The model under review builds one solid part; all positions refer to its coordinate system, in mm. Face numbers are marked on the shaded views. A direction names the side the tool comes from. Give positions to 0.01 mm unless a question says otherwise; leave off trailing zeros. Order: outer loops, then holes, each group sorted by start corner. A loop starts at its lowest first (then second) coordinate and runs counter-clockwise, first axis right, second up.
```python
from build123d import *

# Parameters (mm, degrees)
SKETCH_1_W          = 40
SKETCH_1_H          = 22
SKETCH_1_R          = 4.5
EXTRUDE_1_DEPTH     = 6
CUT_EXTRUDE_2_DEPTH = 4
SKETCH_4_R          = 4.5
CUT_EXTRUDE_3_DEPTH = 7
EXTRUDE_2_DEPTH     = 40
SKETCH_6_W          = 23
SKETCH_6_H          = 13
CUT_EXTRUDE_4_DEPTH = 40
SKETCH_7_R          = 1
CUT_EXTRUDE_5_DEPTH = 40


with BuildPart() as part:
    # 草图1 → 凸台-拉伸1 (new body)
    with BuildSketch(Plane.XY):
        Rectangle(SKETCH_1_W, SKETCH_1_H)
        with BuildLine():
            add(Edge.make_bspline(
                [(3.991210712, -4.387982431), (18, -3.591602336), (18, 0), (18, 3.591602336), (3.991210712, 4.387982431)],
                knots=[4.935981285, 4.935981285, 4.935981285, 6.283185307, 6.283185307, 7.630389329, 7.630389329, 7.630389329], degree=2, weights=[1, 0.781579788, 1, 0.781579788, 1]))
            add(Edge.make_bspline(
                [(3.991210712, 4.387982431), (0, 20.567539049), (-3.991210712, 4.387982431)],
                knots=[5.192517184, 5.192517184, 5.192517184, 7.373853431, 7.373853431, 7.373853431], degree=2, weights=[1, 0.461892887, 1]))
            add(Edge.make_bspline(
                [(-3.991210712, 4.387982431), (-18, 3.591602336), (-18, 0), (-18, -3.591602336), (-3.991210712, -4.387982431)],
                knots=[1.794388632, 1.794388632, 1.794388632, 3.141592654, 3.141592654, 4.488796676, 4.488796676, 4.488796676], degree=2, weights=[1, 0.781579788, 1, 0.781579788, 1]))
            add(Edge.make_bspline(
                [(-3.991210712, -4.387982431), (0, -20.567539049), (3.991210712, -4.387982431)],
                knots=[2.05092453, 2.05092453, 2.05092453, 4.232260777, 4.232260777, 4.232260777], degree=2, weights=[1, 0.461892887, 1]))
        make_face(mode=Mode.SUBTRACT)
        with BuildLine():
            add(Edge.make_bspline(
                [(-3.991210712, -4.387982431), (0, -20.567539049), (3.991210712, -4.387982431)],
                knots=[2.05092453, 2.05092453, 2.05092453, 4.232260777, 4.232260777, 4.232260777], degree=2, weights=[1, 0.461892887, 1]))
            add(Edge.make_bspline(
                [(3.991210712, -4.387982431), (18, -3.591602336), (18, 0), (18, 3.591602336), (3.991210712, 4.387982431)],
                knots=[4.935981285, 4.935981285, 4.935981285, 6.283185307, 6.283185307, 7.630389329, 7.630389329, 7.630389329], degree=2, weights=[1, 0.781579788, 1, 0.781579788, 1]))
            add(Edge.make_bspline(
                [(3.991210712, 4.387982431), (0, 20.567539049), (-3.991210712, 4.387982431)],
                knots=[5.192517184, 5.192517184, 5.192517184, 7.373853431, 7.373853431, 7.373853431], degree=2, weights=[1, 0.461892887, 1]))
            add(Edge.make_bspline(
                [(-3.991210712, 4.387982431), (-18, 3.591602336), (-18, 0), (-18, -3.591602336), (-3.991210712, -4.387982431)],
                knots=[1.794388632, 1.794388632, 1.794388632, 3.141592654, 3.141592654, 4.488796676, 4.488796676, 4.488796676], degree=2, weights=[1, 0.781579788, 1, 0.781579788, 1]))
        make_face()
        Circle(SKETCH_1_R, mode=Mode.SUBTRACT)
        Circle(SKETCH_1_R)
    extrude(amount=EXTRUDE_1_DEPTH)

    # 草图3 → 切除-拉伸2 (cut)
    with BuildSketch(Plane.XY.offset(6)):
        with BuildLine():
            add(Edge.make_bspline(
                [(3.991210712, -4.387982431), (18, -3.591602336), (18, 0), (18, 3.591602336), (3.991210712, 4.387982431)],
                knots=[4.935981285, 4.935981285, 4.935981285, 6.283185307, 6.283185307, 7.630389329, 7.630389329, 7.630389329], degree=2, weights=[1, 0.781579788, 1, 0.781579788, 1]))
            add(Edge.make_bspline(
                [(3.991210712, 4.387982431), (0, 20.567539049), (-3.991210712, 4.387982431)],
                knots=[5.192517184, 5.192517184, 5.192517184, 7.373853431, 7.373853431, 7.373853431], degree=2, weights=[1, 0.461892887, 1]))
            add(Edge.make_bspline(
                [(-3.991210712, 4.387982431), (-18, 3.591602336), (-18, 0), (-18, -3.591602336), (-3.991210712, -4.387982431)],
                knots=[1.794388632, 1.794388632, 1.794388632, 3.141592654, 3.141592654, 4.488796676, 4.488796676, 4.488796676], degree=2, weights=[1, 0.781579788, 1, 0.781579788, 1]))
            add(Edge.make_bspline(
                [(-3.991210712, -4.387982431), (0, -20.567539049), (3.991210712, -4.387982431)],
                knots=[2.05092453, 2.05092453, 2.05092453, 4.232260777, 4.232260777, 4.232260777], degree=2, weights=[1, 0.461892887, 1]))
        make_face()
    extrude(amount=-CUT_EXTRUDE_2_DEPTH, mode=Mode.SUBTRACT)

    # 草图4 → 切除-拉伸3 (cut, through all)
    with BuildSketch(Plane.XY.offset(6)):
        Circle(SKETCH_4_R)
    extrude(amount=-CUT_EXTRUDE_3_DEPTH, mode=Mode.SUBTRACT)

    # 草图5 → 凸台-拉伸2 (add)
    with BuildSketch(Plane.XY.offset(6)):
        Polygon((20, -11), (-20, -11), (-20, -9.5), (-20, 9.5), (-20, 11), (20, 11), (20, 9.5), (-18, 9.5), (-18, -9.5), (20, -9.5), align=None)
    extrude(amount=EXTRUDE_2_DEPTH)

    # 草图6 → 切除-拉伸4 (cut)
    with BuildSketch(Plane.ZY.offset(20)):
        with Locations((23, 0)):
            Rectangle(SKETCH_6_W, SKETCH_6_H)
    extrude(amount=-CUT_EXTRUDE_4_DEPTH, mode=Mode.SUBTRACT)

    # 草图7 → 切除-拉伸5 (cut)
    with BuildSketch(Plane.ZY.offset(20)):
        with Locations((38.5, 0)):
            Circle(SKETCH_7_R)
        with Locations((7.5, 0)):
            Circle(SKETCH_7_R)
    extrude(amount=-CUT_EXTRUDE_5_DEPTH, mode=Mode.SUBTRACT)


solid = part.part
```
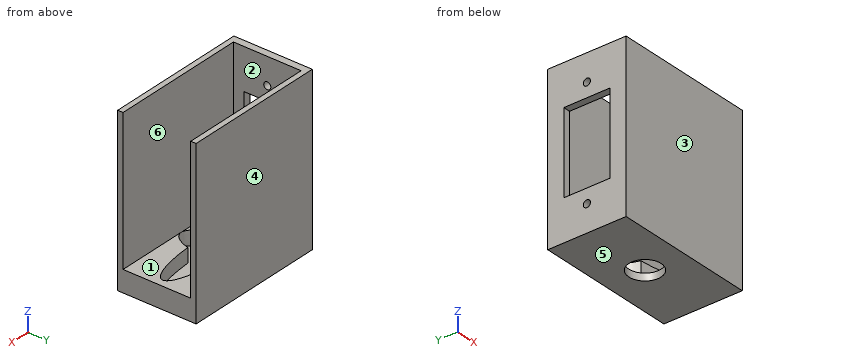
Item 1: Draft analysis for pull direction Y (two halves, no side actions). For the marked faces 1, 2, 3 and 4, state which applies: released by +Y, released by -Y, zero draft, split by the parting line, or undercut.
Values found:
face 1: undercut
face 2: undercut
face 3: released by -Y
face 4: released by +Y
Item 2: Take a section at A-A (z = 19.5). Give the boundary of the cut face in (x, y), and give its area (3 significant figures).
Values found:
outline: (-20, -11) - (20, -11) - (20, -9.5) - (-18, -9.5) - (-18, -6.5) - (-20, -6.5) - close; (-20, 6.5) - (-18, 6.5) - (-18, 9.5) - (20, 9.5) - (20, 11) - (-20, 11) - close
area: 132 mm2
Item 3: Clearance check with flat-ended pins moving along their axes: pin 1 Ø6 at (y, z) = (2, 17.5) entering from -X; pin 2 Ø3 at (x, y) = (-10.5, -4.5) entering from +Z. State where each tip first meets the part, or that it passes through.
Values found:
pin 1: passes through
pin 2: stops at z = 6
Item 4: Take a section at B-B (z = 42). Give the boundary of the cut face in (x, y), and give its area (3 significant figures).
Values found:
outline: (-20, -11) - (20, -11) - (20, -9.5) - (-18, -9.5) - (-18, 9.5) - (20, 9.5) - (20, 11) - (-20, 11) - close
area: 158 mm2
Item 5: For line 1 (Y direction, x = -19.1, z = 7.5); line 2 (Y direction, x = 1, z = 15.5); line 3 (Z direction, x = -5, y = -2.5), list the stretches that pass through material, from the lowest coordinate up.
Values found:
line 1: y = -11 to -1, 1 to 11
line 2: y = -11 to -9.5, 9.5 to 11
line 3: z = 0 to 2
Item 6: For the marked faces 5 and 6, list the 3-axis set-ups (+Z, -Z, +X, -X, +Y, -Y) from which the entire face can be reached by the end or side of a thin tool; tool diameter is ignored.
Values found:
face 5: -Z, +X, -X, +Y, -Y
face 6: +Z, +X
Item 7: Take a section at C-C (y = -3.5). Give the number of separate pieces and of enclosed holes in the cut face, and give its area (3 significant figures).
Values found:
separate pieces: 3
enclosed holes: 0
area: 172 mm2
